CAD build for the part. Positions are in the model's coordinates, mm. Face numbers are marked on the shaded views. A direction names the side the tool comes from. Round coordinates to 2 decimals unless told otherwise and drop trailing zeros. Write each loop counter-clockwise with the first axis right and the second up, starting at its lowest first coordinate (ties: lowest second). Pieces come first, ordered by that corner, then holes. Notation, with made-up numbers: (86, 29) - (140, 29) arc R25 ccw to (140, 45) - close; hole circle Ø8 at (-14, -17.75). An arc over 180 degrees is marked (long way). Use one line per item in the form item = value. Start each with the question number.
Item 1: Band-saw the part on B-B, the plane y = 8. List the corners of the cut face in (x, z), and give its area (3 significant figures).
Item 2: Drill centre lines: L1, parallel to Z at x = 1, y = 8.5; L2, parallel to Z at x = 5.25, y = 0.5; L3, parallel to Y at x = 5, z = -1.5. Where is each one in solid material? Low to high.
Item 3: Pull direction Z, two halves, no side cores. Call the marked faces 1, 2, 3 and 4: +Z half, -Z half, draft (parallel to the pull), parting line (faces both ways), or undercut.
Item 4: Pin check, flat tips, straight feed: pin 1 (5.5 mm diameter, centred on x = 4.5, z = 0, fed in from -Y); pin 2 (10 mm diameter, centred on y = 12.5, z = 1.5, fed in from -X); pin 3 (4 mm diameter, centred on x = -4.5, y = 0.5, fed in from -Z); pin 4 (3 mm diameter, centred on x = 1.5, z = 5, fed in from -Y). Stop position of each tip, or through.
Item 5: Band-saw the part on C-C, the plane z = 0. List the corners of the cut face in (x, y), and give its area (3 significant figures).
Item 6: Band-saw the part on D-D, the plane y = 11.25. List the corners of the cut face in (x, z), and give its area (3 significant figures).
Item 7: Band-saw the part on A-A, the plane x = 0. List the corners of the cut face in (y, z), and give its area (3 significant figures).
Item 8: Tool access for the marked faces 5, 6, 7 and 8: list every direction of +Z, -Z, +X, -X, +Y, -Y with a clear straight run to the whole face (end or side of a thin tool).
from build123d import *

# Parameters (mm, degrees)
BOSS_EXTRUDE1_DEPTH = 2
SKETCH2_R           = 1.55
CUT_EXTRUDE1_DEPTH  = 15.352700094
CHAMFER1_SIZE       = 0.5
SKETCH4_W           = 2
SKETCH4_H           = 14.133755883
CUT_EXTRUDE2_DEPTH  = 6.5
SKETCH5_R           = 1
CUT_EXTRUDE3_DEPTH  = 6.5
SKETCH6_R           = 3
BOSS_EXTRUDE2_DEPTH = 1


with BuildPart() as part:
    # Sketch1 → Boss-Extrude1 (new body)
    with BuildSketch(Plane(origin=(0, 0, 0), x_dir=(1, 0, 0), z_dir=(0, 1, 0))):
        with BuildLine():
            Line((-9, -6.32455532), (-9, 6.32455532))
            ThreePointArc((-9, 6.32455532), (0, 11), (9, 6.32455532))
            Line((9, 6.32455532), (9, -6.32455532))
            ThreePointArc((9, -6.32455532), (0, -11), (-9, -6.32455532))
        make_face()
    extrude(amount=BOSS_EXTRUDE1_DEPTH)

    # Sketch2 → Cut-Extrude1 (cut, through all)
    with BuildSketch(Plane(origin=(0, 2, 0), x_dir=(1, 0, 0), z_dir=(0, 1, 0))):
        with Locations(Location((4.949747468, 4.949747468, 0), (0, 0, 270))):
            Circle(SKETCH2_R)
        with Locations(Location((4.949747468, -4.949747468, 0), (0, 0, 270))):
            Circle(SKETCH2_R)
        with Locations(Location((-4.949747468, -4.949747468, 0), (0, 0, 270))):
            Circle(SKETCH2_R)
        with Locations(Location((-4.949747468, 4.949747468, 0), (0, 0, 270))):
            Circle(SKETCH2_R)
    extrude(amount=-CUT_EXTRUDE1_DEPTH, mode=Mode.SUBTRACT)

    # Chamfer1
    chamfer1_edges = [part.edges().sort_by_distance(p)[0] for p in [
        (0, 2, -11),
        (-4.949747468, 2, -6.499747468),
        (-4.949747468, 2, 3.399747468),
        (4.949747468, 2, 3.399747468),
        (4.949747468, 2, -6.499747468),
        (0, 2, 11),
    ]]
    chamfer(chamfer1_edges, length=CHAMFER1_SIZE)

    # Sketch3 → Revolve1 (revolve)
    with BuildSketch(Plane.XY):
        with BuildLine():
            Line((0, 2), (4, 2))
            Line((4, 2), (4, 12))
            ThreePointArc((4, 12), (2.828427125, 14.828427125), (0, 16))
            Line((0, 16), (0, 2))
        make_face()
    revolve(axis=Axis((0, 2, 0), (0, 1, 0)))

    # Sketch4 → Cut-Extrude2 (cut, symmetric)
    with BuildSketch(Plane(origin=(0, 0, 0), x_dir=(0, 0, -1), z_dir=(1, 0, 0))):
        with Locations((0, 12.566877942)):
            Rectangle(SKETCH4_W, SKETCH4_H)
    extrude(amount=CUT_EXTRUDE2_DEPTH, both=True, mode=Mode.SUBTRACT)

    # Sketch5 → Cut-Extrude3 (cut, symmetric)
    with BuildSketch(Plane.XY):
        with Locations((0, 8)):
            Circle(SKETCH5_R)
    extrude(amount=CUT_EXTRUDE3_DEPTH, both=True, mode=Mode.SUBTRACT)

    # Sketch6 → Boss-Extrude2 (add)
    with BuildSketch(Plane.XZ):
        with Locations(Location((0, 0, 0), (0, 0, 90))):
            Circle(SKETCH6_R)
    extrude(amount=BOSS_EXTRUDE2_DEPTH)


solid = part.part
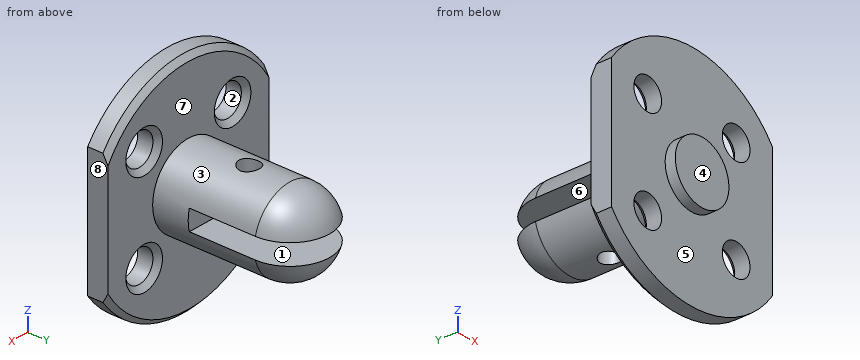
Determined:
q1.outline = (-3.87, -1) arc R4 ccw to (-1, -3.87) - (-1, -1) - close; (-3.87, 1) - (-1, 1) - (-1, 3.87) arc R4 ccw to start; (1, -3.87) arc R4 ccw to (3.87, -1) - (1, -1) - close; (1, 1) - (3.87, 1) arc R4 ccw to (1, 3.87) - close
q1.area = 22.6 mm²
q2.L1 = -3.87 to -1, 1 to 3.87
q2.L2 = -9.67 to -6.47, -3.43 to 3.43, 6.47 to 9.67
q2.L3 = 0 to 2
q3.face_1 = undercut
q3.face_2 = undercut
q3.face_3 = parting line
q3.face_4 = draft
q4.pin_1 = -1
q4.pin_2 = -3.87
q4.pin_3 = -10.71
q4.pin_4 = 0
q5.outline = (-9, 0) - (-3, 0) - (-3, -1) - (3, -1) - (3, 0) - (9, 0) - (9, 2) - (4, 2) - (4, 5.5) - (-4, 5.5) - (-4, 2) - (-9, 2) - close
q5.area = 70.0 mm²
q6.outline = (-3.87, -1) arc R4 ccw to (3.87, -1) - close; (-3.87, 1) - (3.87, 1) arc R4 ccw to start
q6.area = 34.4 mm²
q7.outline = (-1, -3) - (0, -3) - (0, -11) - (1.5, -11) - (2, -10.5) - (2, -4) - (7, -4) - (7, -1) - (5.5, -1) - (5.5, 1) - (7, 1) - (7, 4) - (2, 4) - (2, 10.5) - (1.5, 11) - (0, 11) - (0, 3) - (-1, 3) - close; (9, -4) - (12, -4) arc R4 ccw to (15.87, -1) - (9, -1) - close; (9, 1) - (15.87, 1) arc R4 ccw to (12, 4) - (9, 4) - close
q7.area = 122 mm²
q8.face_5 = -Y
q8.face_6 = +X, -X, +Y
q8.face_7 = +Y
q8.face_8 = +Z, -Z, +X, +Y, -Y
